from build123d import *

# Parameters (mm, degrees)
ESQUISSE1_R        = 2.5
ESQUISSE1_R_2      = 1.75
BOSS_EXTRU_1_DEPTH = 2


with BuildPart() as part:
    # Esquisse1 → Boss.-Extru.1 (new body)
    with BuildSketch(Plane.XY):
        with BuildLine():
            Line((-201.77541219, 13.663200047), (17.971945957, -34.670003728))
            ThreePointArc((17.971945957, -34.670003728), (21.739530729, -33.99920873), (23.929291778, -30.860800298))
            Line((23.929291778, -30.860800298), (72.262495553, 188.88655785))
            ThreePointArc((72.262495553, 188.88655785), (71.591700555, 192.654142622), (68.453292123, 194.843903671))
            Line((68.453292123, 194.843903671), (-151.294066025, 243.177107446))
            ThreePointArc((-151.294066025, 243.177107446), (-155.061650796, 242.506312448), (-157.251411845, 239.367904015))
            Line((-157.251411845, 239.367904015), (-205.584615621, 19.620545868))
            ThreePointArc((-205.584615621, 19.620545868), (-204.913820623, 15.852961096), (-201.77541219, 13.663200047))
        make_face()
        with Locations((-133.322120067, 208.507103718)):
            Circle(ESQUISSE1_R, mode=Mode.SUBTRACT)
        with Locations((-170.914611893, 37.592491825)):
            Circle(ESQUISSE1_R, mode=Mode.SUBTRACT)
        Circle(ESQUISSE1_R, mode=Mode.SUBTRACT)
        with Locations((-100.0322124, 88.043731079)):
            Circle(ESQUISSE1_R_2, mode=Mode.SUBTRACT)
        with Locations((37.592491825, 170.914611893)):
            Circle(ESQUISSE1_R, mode=Mode.SUBTRACT)
        with Locations((-86.359043449, 85.036331733)):
            Circle(ESQUISSE1_R_2, mode=Mode.SUBTRACT)
        with Locations((-76.477588455, 129.962458287)):
            Circle(ESQUISSE1_R_2, mode=Mode.SUBTRACT)
        with Locations((-90.150757406, 132.969857633)):
            Circle(ESQUISSE1_R_2, mode=Mode.SUBTRACT)
    extrude(amount=BOSS_EXTRU_1_DEPTH)


solid = part.part
Can you work these out from the model? Positions are in its coordinate system, mm. Round coordinates to 2 decimals unless told otherwise and drop trailing zeros. Order: outer loops, then holes, each group sorted by start corner. A loop starts at its lowest first (then second) coordinate and runs counter-clockwise, first axis right, second up. Notation, with made-up numbers: M 57,52.25 L 101,52.25 A21 cw 101,59.25 Z; hole C 77.25,86.5 d6. An arc over 180 degrees is marked long. Use a Markdown table: item, result.
1) Imagine slicing it at B-B (y = 104.5). List the corners of the cut face in (x, z) for me, then the cut area to 3 significant figures.
Geometry says:
| item | result |
|---|---|
| outline | M -186.92,0 L 53.7,0 L 53.7,2 L -186.92,2 Z |
| area | 481 mm² |
2) Imagine slicing it at C-C (x = -177.5). List the corners of the cut face in (y, z) for me.
Geometry says:
| item | result |
|---|---|
| outline | M 8.32,0 L 147.31,0 L 147.31,2 L 8.32,2 Z |
3) If I drill on line 1 along X through (y, z) = (131.5, 1.45); line 2 along X through (y, z) = (37.5, 0.75); line 3 along Y through (x, z) = (-148, 0.9), over which ranges is the centre line in solid material (lowest first)?
Geometry says:
| item | result |
|---|---|
| line 1 | x = -180.98 to -91.1, -89.2 to -77.31, -75.64 to 59.64 |
| line 2 | x = -201.65 to -173.41, -168.42 to 38.97 |
| line 3 | y = 1.84 to 242.45 |
4) Imagine slicing it at A-A (z = 0.8). Give the number of separate pieces and of enclosed holes in the cut face, then the cut area to 3 significant figures.
Geometry says:
| item | result |
|---|---|
| separate pieces | 1 |
| enclosed holes | 8 |
| area | 55,100 mm² |
